```python
from build123d import *

# Parameters (mm, degrees)
BOSS_EXTRU_1_DEPTH      = 3
BOSS_EXTRU_2_DEPTH      = 20
ESQUISSE4_W             = 14.470789164
ESQUISSE4_H             = 3
BOSS_EXTRU_3_DEPTH      = 20
CONG_1_R                = 10
ESQUISSE5_R             = 2.6
ENL_V_MAT_EXTRU_1_DEPTH = 20
ESQUISSE6_R             = 2.6
ENL_V_MAT_EXTRU_2_DEPTH = 20
ESQUISSE7_R             = 2.6
ENL_V_MAT_EXTRU_3_DEPTH = 20


with BuildPart() as part:
    # Esquisse1 → Boss.-Extru.1 (new body)
    with BuildSketch(Plane.XY):
        Polygon((-44.709210836, 492.3), (-44.709210836, 472.3), (-64.709210836, 472.3), (-59.901201413, 492.3), align=None)
    extrude(amount=BOSS_EXTRU_1_DEPTH)

    # Esquisse3 → Boss.-Extru.2 (add)
    with BuildSketch(Plane.XY.offset(3)):
        Polygon((-59.901201413, 492.3), (-64.709210836, 472.3), (-61.709210836, 472.3), (-56.901201413, 492.3), align=None)
    extrude(amount=BOSS_EXTRU_2_DEPTH)

    # Esquisse4 → Boss.-Extru.3 (add)
    with BuildSketch(Plane.XY.offset(3)):
        with Locations((-51.944605418, 490.8)):
            Rectangle(ESQUISSE4_W, ESQUISSE4_H)
    extrude(amount=BOSS_EXTRU_3_DEPTH)

    # Congé1
    cong_1_edges = [part.edges().sort_by_distance(p)[0] for p in [
        (-63.209210836, 472.3, 23),
        (-44.709210836, 490.8, 23),
        (-44.709210836, 472.3, 1.5),
    ]]
    fillet(cong_1_edges, radius=CONG_1_R)

    # Esquisse5 → Enlèv. mat.-Extru.1 (cut)
    with BuildSketch(Plane.XY.offset(3)):
        with Locations((-51.165806832, 479.3)):
            Circle(ESQUISSE5_R)
    extrude(amount=-ENL_V_MAT_EXTRU_1_DEPTH, mode=Mode.SUBTRACT)

    # Esquisse6 → Enlèv. mat.-Extru.2 (cut)
    with BuildSketch(Plane.XZ.offset(-489.3)):
        with Locations(Location((-51.165806832, 13, 0), (0, 0, 270))):
            Circle(ESQUISSE6_R)
    extrude(amount=-ENL_V_MAT_EXTRU_2_DEPTH, mode=Mode.SUBTRACT)

    # Esquisse7 → Enlèv. mat.-Extru.3 (cut)
    with BuildSketch(Plane(origin=(-165.675566954, 39.828484352, 0), x_dir=(0, 0, -1), z_dir=(0.9722988712431988, -0.23374110673820636, 0))):
        with Locations(Location((-13, 453.53494557, 0), (0, 0, 90))):
            Circle(ESQUISSE7_R)
    extrude(amount=-ENL_V_MAT_EXTRU_3_DEPTH, mode=Mode.SUBTRACT)


solid = part.part
```
Could you check a few things on this model? Use its own coordinates, in mm. A direction names the side the tool comes from. Round coordinates to 2 decimals unless told otherwise and drop trailing zeros. Loops run counter-clockwise (first coordinate to the right, second up) from the corner with the lowest first, then second, coordinate; pieces in that order, holes last.
Q1. I want a section at A-A (x = -55.25). Write out the boundary of the cut face in (y, z).
Q2. I want a section at C-C (z = 5.25). Write out the boundary of the cut face in (x, y).
Q3. On a 3-axis mill with a long thin cutter (end or side, diameter ignored), from which of +Z, -Z, +X, -X, +Y, -Y can I reach the whole of each face in a straight line? I mean faces 1 (the flat face through (-52.7, 489.3, 10.6)), 2 (the cylindrical face through (-47.56, 475.31, 1.52)). Say none if no direction works.
Q4. Please list where these lines run through material, in increasing order: L1, parallel to Z at x = -56.25, y = 481.75; L2, parallel to Y at x = -48.75, z = 16.75; L3, parallel to X at y = 479.3, z = 1.65.
Q5. Thinking about a two-plate mould opening in Y: for faces 3 (the flat face through (-62, 472.3, 5)), 4 (the cylindrical face through (-61.67, 478.61, 13.11)), 5 (the flat face through (-53, 483, 3)), which applies, pulls with the +Y half, pulls with the -Y half, needs draft (parallel to the pull), parting line crosses it, or undercut?
Q6. For P1, Ø12, axis at x = -47, z = 8, coming from the -Y side; P2, Ø5, axis at x = -55.5, y = 478.5, coming from the +Z side; P3, Ø4, axis at y = 480.5, z = 8.5, coming from the +X side, each with a flat end and sliding along its axis, tell me the tip position at first contact or that it passes through.
Q7. I want a section at B-B (y = 479.3). Give the number of separate pieces and of enclosed holes in the cut face, and give its area (3 significant figures).
Answer below:
1. outline: (472.3, 0) - (492.3, 0) - (492.3, 23) - (489.3, 23) - (489.3, 3) - (472.3, 3) - close
2. outline: (-64.71, 472.3) - (-61.71, 472.3) - (-57.62, 489.3) - (-44.71, 489.3) - (-44.71, 492.3) - (-59.9, 492.3) - close
3. face 1: +Z, +X, -Y
3. face 2: +Z, -Z, +X, -Y
4. L1: z = 0 to 3
4. L2: y = 489.3 to 492.3
4. L3: x = -63.03 to -53.77, -48.57 to -45.17
5. face 3: pulls with the -Y half
5. face 4: undercut
5. face 5: needs draft
6. P1: stops at y = 473.32
6. P2: stops at z = 3
6. P3: stops at x = -59.26
7. separate pieces: 3
7. enclosed holes: 0
7. area: 86.0 mm2
